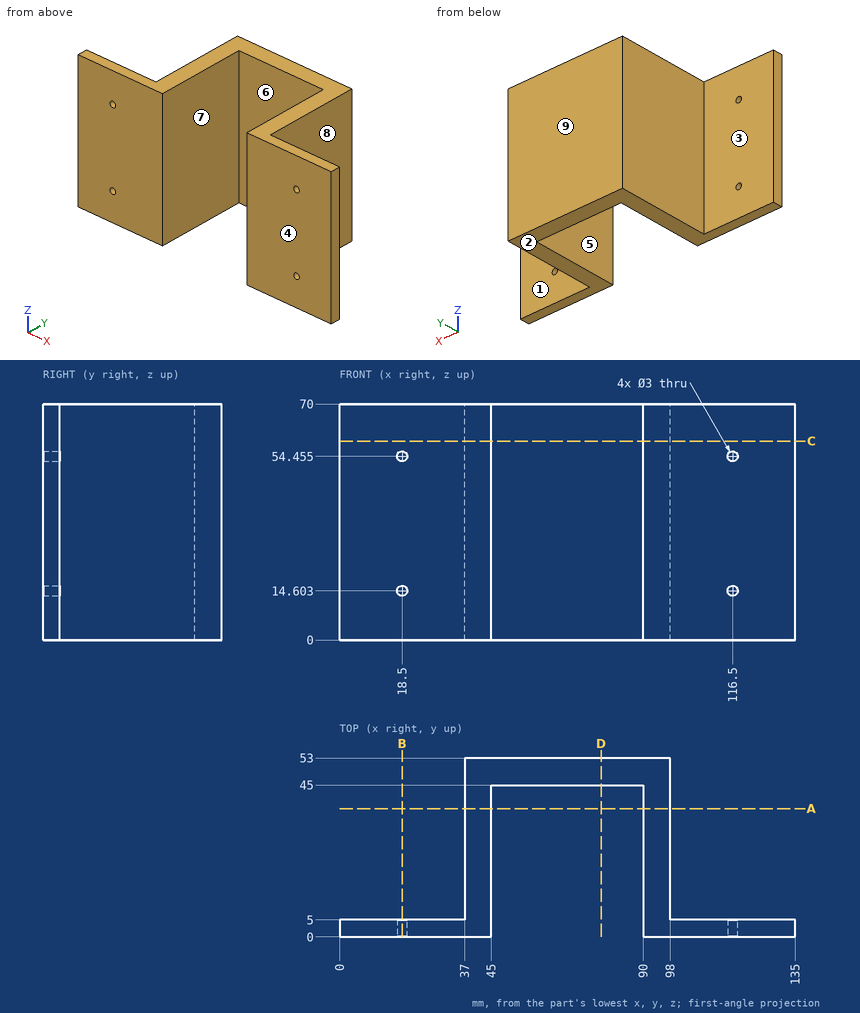
Source: three-view drawing plus pictorial views. Frame: mm from the lowest corner of the part. A direction names the side the tool comes from. Coordinates: 2 decimals unless noted, no trailing zeros. Loops run counter-clockwise (first coordinate to the right, second up) from the corner with the lowest first, then second, coordinate; pieces in that order, holes last. Notation, with made-up numbers: (-35.5, 46.25) - (-16.5, 46.25) arc R24 ccw to (-16.5, 61.25) - close; hole circle Ø6 at (89, -17.75). An arc over 180 degrees is marked (long way). Answer in a Markdown table with one row per item. Add a question column.
Item 1: Contact query for flat-ended pins moving along their axis: P1, Ø1, axis at y = 24.5, z = 61, coming from the +X side; P2, Ø6, axis at y = 42, z = 32, coming from the -X side; P3, Ø2.5, axis at x = 116.5, z = 54.46, coming from the +Y side; P4, Ø11, axis at x = 122.5, z = 31.5, coming from the +Y side. Output: stop coordinate, or through.
Item 2: Access query for the marked faces 1, 2, 3, 4 and 5. Directions: +Z, -Z, +X, -X, +Y, -Y. A direction counts if a zero-diameter tool reaches every point of the face in a straight line with its end or side. Return the directions, or none.
Item 3: Section query B-B on x = 18.5. Return the cut outline in (y, z) (1 decimal).
Item 4: Mould query, pull axis X, two halves, no side actions, for the marked faces 6, 7, 8 and 9. Classes: released by +X, released by -X, zero draft, split by the parting line, or undercut.
Item 5: Section query C-C on z = 59. Return the cut outline in (x, y), then the cut area to 3 significant figures.
Item 6: Section query D-D on x = 77.5. Return the cut outline in (y, z).
Item 7: Section query A-A on y = 38. Return the cut outline in (x, z), then the cut area to 3 significant figures.
Item 8: Line query: line 1 along Z through (x, y) = (116.5, 1.2) (1 decimal); line 2 along X through (y, z) = (32, 23.5); line 3 along Z through (x, y) = (116, 1). Output: solid intervals per line, ascending. Write a range as [from, to].
Recorded:
| question | item | result |
|---|---|---|
| 1 | P1 | x = 98 |
| 1 | P2 | x = 37 |
| 1 | P3 | through |
| 1 | P4 | y = 5 |
| 2 | face 1 | +Z, -Z, +X, +Y |
| 2 | face 2 | -Z, +X, -X, +Y, -Y |
| 2 | face 3 | +Z, -Z, -X, +Y |
| 2 | face 4 | +Z, -Z, +X, -X, -Y |
| 2 | face 5 | +Z, -Z, -Y |
| 3 | outline | (0, 0) - (5, 0) - (5, 13.1) - (0, 13.1) - close; (0, 16.1) - (5, 16.1) - (5, 53) - (0, 53) - close; (0, 56) - (5, 56) - (5, 70) - (0, 70) - close |
| 4 | face 6 | undercut |
| 4 | face 7 | undercut |
| 4 | face 8 | released by +X |
| 4 | face 9 | zero draft |
| 5 | outline | (0, 0) - (45, 0) - (45, 45) - (90, 45) - (90, 0) - (135, 0) - (135, 5) - (98, 5) - (98, 53) - (37, 53) - (37, 5) - (0, 5) - close |
| 5 | area | 1,580 mm^2 |
| 6 | outline | (45, 0) - (53, 0) - (53, 70) - (45, 70) - close |
| 7 | outline | (37, 0) - (45, 0) - (45, 70) - (37, 70) - close; (90, 0) - (98, 0) - (98, 70) - (90, 70) - close |
| 7 | area | 1,120 mm^2 |
| 8 | line 1 | [0, 13.1], [16.1, 53], [56, 70] |
| 8 | line 2 | [37, 45], [90, 98] |
| 8 | line 3 | [0, 13.19], [16.02, 53.04], [55.87, 70] |
